Here's how the part is built. I have some questions about the finished solid (model axes, mm). Round coordinates to 2 decimals unless told otherwise and drop trailing zeros. Order: outer loops, then holes, each group sorted by start corner. A loop starts at its lowest first (then second) coordinate and runs counter-clockwise, first axis right, second up. Notation, with made-up numbers: (53, -26.75) - (66, -26.75) arc R8 cw to (66, -20.75) - close; hole circle Ø5 at (-36, -6.75). An arc over 180 degrees is marked (long way). Answer as a JSON object with one key per item and string values.
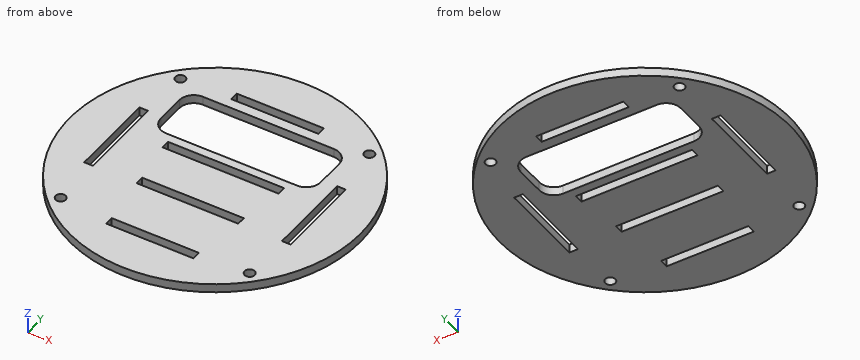
```python
from build123d import *

# Parameters (mm, degrees)
SKETCH_1_R          = 50
EXTRUDE_1_DEPTH     = 3
SKETCH_2_W          = 30
SKETCH_2_H          = 3
SKETCH_2_W_2        = 35
SKETCH_2_W_3        = 40
CUT_EXTRUDE_1_DEPTH = 8
CUT_EXTRUDE_2_DEPTH = 10
SKETCH_4_W          = 2.995674625
SKETCH_4_H          = 30
CUT_EXTRUDE_3_DEPTH = 10
SKETCH_5_R          = 1.75
CUT_EXTRUDE_4_DEPTH = 10


with BuildPart() as part:
    # Эскиз1 → Бобышка-Вытянуть1 (new body)
    with BuildSketch(Plane.XY):
        Circle(SKETCH_1_R)
    extrude(amount=EXTRUDE_1_DEPTH)

    # Эскиз2 → Вырез-Вытянуть1 (cut)
    with BuildSketch(Plane.XY.offset(3)):
        with Locations((0, -34)):
            Rectangle(SKETCH_2_W, SKETCH_2_H)
        with Locations((0, -13.5)):
            Rectangle(SKETCH_2_W_2, SKETCH_2_H)
        with Locations((0, 4.5)):
            Rectangle(SKETCH_2_W_3, SKETCH_2_H)
        with Locations((0, 34)):
            Rectangle(SKETCH_2_W, SKETCH_2_H)
    extrude(amount=-CUT_EXTRUDE_1_DEPTH, mode=Mode.SUBTRACT)

    # Эскиз3 → Вырез-Вытянуть2 (cut)
    with BuildSketch(Plane(origin=(0, 0, 0), x_dir=(-1, 0, 0), z_dir=(0, 0, -1))):
        with BuildLine():
            Line((-22.5, 29), (22.5, 29))
            ThreePointArc((22.5, 29), (26.035533906, 27.535533906), (27.5, 24))
            Line((27.5, 24), (27.5, 14))
            ThreePointArc((27.5, 14), (26.035533906, 10.464466094), (22.5, 9))
            Line((22.5, 9), (-22.5, 9))
            ThreePointArc((-22.5, 9), (-26.035533906, 10.464466094), (-27.5, 14))
            Line((-27.5, 14), (-27.5, 24))
            ThreePointArc((-27.5, 24), (-26.035533906, 27.535533906), (-22.5, 29))
        make_face()
    extrude(amount=-CUT_EXTRUDE_2_DEPTH, mode=Mode.SUBTRACT)

    # Эскиз4 → Вырез-Вытянуть3 (cut)
    with BuildSketch(Plane(origin=(0, 0, 0), x_dir=(-1, 0, 0), z_dir=(0, 0, -1))):
        with Locations((-33.997837312, 0)):
            Rectangle(SKETCH_4_W, SKETCH_4_H)
        with Locations((33.997837312, 0)):
            Rectangle(SKETCH_4_W, SKETCH_4_H)
    extrude(amount=-CUT_EXTRUDE_3_DEPTH, mode=Mode.SUBTRACT)

    # Эскиз5 → Вырез-Вытянуть4 (cut)
    with BuildSketch(Plane.XY.offset(3)):
        with Locations((-32.5, 32.5)):
            Circle(SKETCH_5_R)
        with Locations((32.5, 32.5)):
            Circle(SKETCH_5_R)
        with Locations((32.5, -32.5)):
            Circle(SKETCH_5_R)
        with Locations((-32.5, -32.5)):
            Circle(SKETCH_5_R)
    extrude(amount=-CUT_EXTRUDE_4_DEPTH, mode=Mode.SUBTRACT)


solid = part.part
```
1. Imagine slicing it at B-B (x = 0). List the corners of the cut face in (y, z) for me.
Responses:
{"outline": "(-50, 0) - (-35.5, 0) - (-35.5, 3) - (-50, 3) - close; (-32.5, 0) - (-15, 0) - (-15, 3) - (-32.5, 3) - close; (-12, 0) - (3, 0) - (3, 3) - (-12, 3) - close; (6, 0) - (9, 0) - (9, 3) - (6, 3) - close; (29, 0) - (32.5, 0) - (32.5, 3) - (29, 3) - close; (35.5, 0) - (50, 0) - (50, 3) - (35.5, 3) - close"}
2. Imagine slicing it at D-D (z = 2.05). Give the number of separate pieces and of enclosed holes in the cut face, plus the area to 3 significant figures.
Responses:
{"separate pieces": "1", "enclosed holes": "11", "area": "6,150 mm2"}
3. If I drill on L1, parallel to Y at x = 14.5, z = 0.8; L2, parallel to Y at x = 13, z = 2.8; L3, parallel to X at y = 11, z = 1.9 (3 decimals), over which ranges is the centre line in solid material (lowest first)? Write a range as [from, to].
Responses:
{"L1": "[-47.85, -35.5], [-32.5, -15], [-12, 3], [6, 9], [29, 32.5], [35.5, 47.85]", "L2": "[-48.28, -35.5], [-32.5, -15], [-12, 3], [6, 9], [29, 32.5], [35.5, 48.28]", "L3": "[-48.775, -35.496], [-32.5, -26.5], [26.5, 32.5], [35.496, 48.775]"}
4. Imagine slicing it at C-C (x = 26). List the corners of the cut face in (y, z) for me, plus the area to 3 significant figures.
Responses:
{"outline": "(-42.71, 0) - (10.43, 0) - (10.43, 3) - (-42.71, 3) - close; (27.57, 0) - (42.71, 0) - (42.71, 3) - (27.57, 3) - close", "area": "205 mm2"}
5. Imagine slicing it at A-A (y = 0). List the corners of the cut face in (x, z) for me, plus the area to 3 significant figures.
Responses:
{"outline": "(-50, 0) - (-35.5, 0) - (-35.5, 3) - (-50, 3) - close; (-32.5, 0) - (32.5, 0) - (32.5, 3) - (-32.5, 3) - close; (35.5, 0) - (50, 0) - (50, 3) - (35.5, 3) - close", "area": "282 mm2"}
6. For P1, Ø1.5, axis at x = -33.5, z = 1, coming from the +Y side; P2, Ø1.5, axis at y = -33.5, z = 1.5, coming from the +X side; P3, Ø1, axis at y = 7, z = 2, coming from the +X side, each with a flat end and sliding along its axis, tell me the tip position at first contact or that it passes through.
Responses:
{"P1": "y = 37.78", "P2": "x = 37.78", "P3": "x = 49.58"}
